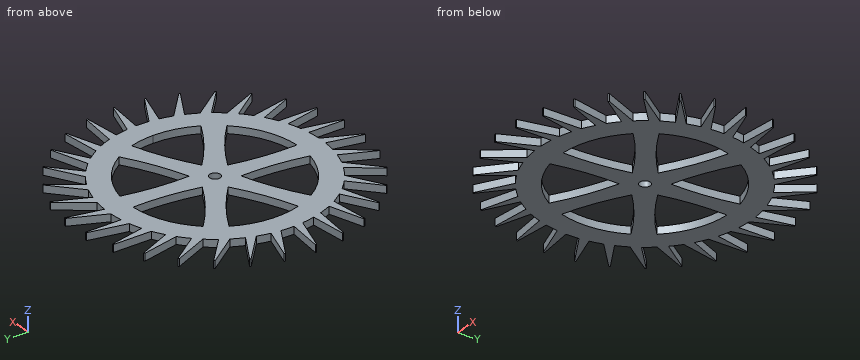
from build123d import *

# Parameters (mm, degrees)
SKETCH1_R           = 63.5
BOSS_EXTRUDE1_DEPTH = 4.445
BOSS_EXTRUDE2_START = -4.445
BOSS_EXTRUDE2_DEPTH = 4.445
CIRPATTERN1_COUNT   = 30
SKETCH3_R           = 3.175
CUT_EXTRUDE1_DEPTH  = 120.591712413
CUT_EXTRUDE2_DEPTH  = 120.591712413


with BuildPart() as part:
    # Sketch1 → Boss-Extrude1 (new body)
    with BuildSketch(Plane.XY):
        Circle(SKETCH1_R)
    extrude(amount=BOSS_EXTRUDE1_DEPTH)

    # Sketch2 → Boss-Extrude2 (add)
    with BuildSketch(Plane.XY.offset(4.445).offset(BOSS_EXTRUDE2_START)):
        with BuildLine():
            Line((9.626690277, 84.117518638), (0, 63.5))
            ThreePointArc((0, 63.5), (2.779385353, 63.439144202), (5.553443409, 63.256693451))
            Line((5.553443409, 63.256693451), (10.360378235, 84.030308047))
            Line((10.360378235, 84.030308047), (9.626690277, 84.117518638))
        make_face()
    boss_extrude2 = extrude(amount=BOSS_EXTRUDE2_DEPTH)

    # CirPattern1: Boss-Extrude2 ×30 about axis
    cirpattern1_axis = Axis((0, 0, 0), (0, 0, 1))
    for i in range(1, CIRPATTERN1_COUNT):
        add(boss_extrude2.rotate(cirpattern1_axis, i * 360 / CIRPATTERN1_COUNT))

    # Sketch3 → Cut-Extrude1 (cut, through all)
    with BuildSketch(Plane.XY.offset(4.445)):
        Circle(SKETCH3_R)
    extrude(amount=-CUT_EXTRUDE1_DEPTH, mode=Mode.SUBTRACT)

    # Sketch4 → Cut-Extrude2 (cut, through all)
    with BuildSketch(Plane.XY.offset(4.445)):
        with BuildLine():
            Line((-5.165555367, 11.602027312), (-1.046816164, 50.789213185))
            ThreePointArc((-1.046816164, 50.789213185), (-20.662221468, 46.408109248), (-37.043284234, 34.76255303))
            ThreePointArc((-37.043284234, 34.76255303), (-21.850907071, 22.154838588), (-5.165555367, 11.602027312))
        make_face()
        with BuildLine():
            ThreePointArc((-48.626896141, -14.699148671), (-30.11210657, -7.846021325), (-12.630428071, 1.327511483))
            ThreePointArc((-12.630428071, 1.327511483), (-27.822805234, 13.935225925), (-44.508156938, 24.488037201))
            ThreePointArc((-44.508156938, 24.488037201), (-50.521712285, 5.310045934), (-48.626896141, -14.699148671))
        make_face()
        with BuildLine():
            ThreePointArc((-11.583611907, -49.461701701), (-8.261199499, -30.000859913), (-7.464872704, -10.274515829))
            ThreePointArc((-7.464872704, -10.274515829), (-25.979662276, -17.127643175), (-43.461340774, -26.301175983))
            ThreePointArc((-43.461340774, -26.301175983), (-29.859490816, -41.098063314), (-11.583611907, -49.461701701))
        make_face()
        with BuildLine():
            ThreePointArc((37.043284234, -34.76255303), (21.850907071, -22.154838588), (5.165555367, -11.602027312))
            ThreePointArc((5.165555367, -11.602027312), (1.843142958, -31.0628691), (1.046816164, -50.789213185))
            ThreePointArc((1.046816164, -50.789213185), (20.662221468, -46.408109248), (37.043284234, -34.76255303))
        make_face()
        with BuildLine():
            ThreePointArc((48.626896141, 14.699148671), (30.11210657, 7.846021325), (12.630428071, -1.327511483))
            ThreePointArc((12.630428071, -1.327511483), (27.822805234, -13.935225925), (44.508156938, -24.488037201))
            ThreePointArc((44.508156938, -24.488037201), (49.201902262, -12.64170929), (50.8, 0))
            ThreePointArc((50.8, 0), (50.253787539, 7.429457451), (48.626896141, 14.699148671))
        make_face()
        with BuildLine():
            ThreePointArc((43.461340774, 26.301175983), (29.859490816, 41.098063314), (11.583611907, 49.461701701))
            Line((11.583611907, 49.461701701), (7.464872704, 10.274515829))
            ThreePointArc((7.464872704, 10.274515829), (25.979662276, 17.127643175), (43.461340774, 26.301175983))
        make_face()
        with BuildLine():
            Line((-1.046816164, 50.789213185), (-5.165555367, 11.602027312))
            ThreePointArc((-5.165555367, 11.602027312), (-1.843142958, 31.0628691), (-1.046816164, 50.789213185))
        make_face()
        with BuildLine():
            ThreePointArc((7.464872704, 10.274515829), (8.261199499, 30.000859913), (11.583611907, 49.461701701))
            Line((11.583611907, 49.461701701), (7.464872704, 10.274515829))
        make_face()
    extrude(amount=-CUT_EXTRUDE2_DEPTH, mode=Mode.SUBTRACT)


solid = part.part
Verification items for the finished model (mm, model axes). Round coordinates to 2 decimals unless told otherwise and drop trailing zeros. Order: outer loops, then holes, each group sorted by start corner. A loop starts at its lowest first (then second) coordinate and runs counter-clockwise, first axis right, second up. Notation, with made-up numbers: (60, 55.5) -> (85, 55.5) arc R18 cw to (85, 67.5) -> close; hole circle Ø5 at (24.25, 17.5). An arc over 180 degrees is marked (long way). Put each result on its own line as item: value.
1) Section check A-A (x = -16). Record the cut outline in (y, z) (3 decimals), then the cut area to 3 significant figures.
Final values:
outline: (-65.821, 0) -> (-48.215, 0) -> (-48.215, 4.445) -> (-65.821, 4.445) -> close; (-13.098, 0) -> (-0.669, 0) -> (-0.669, 4.445) -> (-13.098, 4.445) -> close; (4.418, 0) -> (18.108, 0) -> (18.108, 4.445) -> (4.418, 4.445) -> close; (48.215, 0) -> (61.451, 0) -> (61.451, 4.445) -> (48.215, 4.445) -> close
area: 253 mm^2
2) Depth check by flat-ended pin: pin 1 (12 mm diameter, centred on x = -41, y = 56, fed in from -Z); pin 2 (4 mm diameter, centred on x = 21.5, y = 18.5, fed in from +Z); pin 3 (1.5 mm diameter, centred on x = -0.5, z = 3, fed in from +Y); pin 4 (1.5 mm diameter, centred on x = 38.5, z = 1.5, fed in from -Y). Enter the tip coordinate at first touch or a pass-through.
Final values:
pin 1: stops at z = 0
pin 2: passes through
pin 3: stops at y = 64.04
pin 4: stops at y = -69.92
3) Section check B-B (y = 68). Record the cut outline in (x, z) (3 decimals), then the cut area to 3 significant figures.
Final values:
outline: (-40.548, 0) -> (-38.436, 0) -> (-38.436, 4.445) -> (-40.548, 4.445) -> close; (-25.648, 0) -> (-22.197, 0) -> (-22.197, 4.445) -> (-25.648, 4.445) -> close; (-11.84, 0) -> (-7.63, 0) -> (-7.63, 4.445) -> (-11.84, 4.445) -> close; (2.101, 0) -> (6.651, 0) -> (6.651, 4.445) -> (2.101, 4.445) -> close; (17.644, 0) -> (21.983, 0) -> (21.983, 4.445) -> (17.644, 4.445) -> close; (37.331, 0) -> (40.209, 0) -> (40.209, 4.445) -> (37.331, 4.445) -> close
area: 95.7 mm^2
4) Section check C-C (z = 2.7). Give the number of separate pieces and of enclosed holes in the cut face, then the cut area to 3 significant figures.
Final values:
separate pieces: 1
enclosed holes: 7
area: 9,550 mm^2
5) Material ranges on line 1 (Y direction, x = 0, z = 3.35) (3 decimals); line 2 (Y direction, x = -19.5, z = 0.9); line 3 (Y direction, x = -69, z = 2), recorded low to high.
Final values:
line 1: y = -63.5 to -3.175, 3.175 to 63.5
line 2: y = -70.46 to -62.68, -60.43 to -46.91, -14.42 to -2.62, 7.44 to 20.48, 46.91 to 60.43
line 3: y = -49.07 to -48.32, -32.97 to -30.31, -18.56 to -14.89, -4.62 to -0.41, 10.16 to 14.44, 27.66 to 31.18
